Autodesk Inventor part; units mm, degrees
ref_plane "YZ Plane" through (0, 0, 0) normal (1, 0, 0) x (0, 1, 0)
ref_plane "XZ Plane" through (0, 0, 0) normal (0, 1, 0) x (-1, 0, 0)
ref_plane "XY Plane" through (0, 0, 0) normal (0, 0, 1) x (1, 0, 0)
sketch "스케치1" plane through (0, 0, 0) normal (0, 0, 1) x (1, 0, 0)
  line L0 (14.1048, -8.184) -> (-14.1048, -8.184)
  line L1 (-14.1048, -8.184) -> (-14.1048, 8.184)
  line L2 (-14.1048, 8.184) -> (14.1048, 8.184)
  line L3 (14.1048, 8.184) -> (14.1048, -8.184)
  line L4 (14.1048, -8.184) -> (-14.1048, 8.184) construction
  line L5 (-14.1048, -8.184) -> (14.1048, 8.184) construction
  point P0 (0, 0)
extrude "돌출1" add sketch "스케치1" along normal blind 20
sketch "스케치2" plane through (-14.1048, 8.184, 0) normal (0, 1, 0) x (1, 0, 0)
  line L0 (0, -20) -> (28.2096, -20)
  line L1 (28.2096, 0) -> (0, 0)
  line L2 (6.0629, -20) -> (28.2096, -20)
  line L3 (28.2096, -20) -> (28.2096, 0)
  line L4 (28.2096, 0) -> (6.0629, 0)
  line L5 (6.0629, 0) -> (6.0629, -20)
  point P0 (14.1048, 0)
extrude "돌출2" cut sketch "스케치2" against normal blind 8
sketch "스케치3" plane through (-14.1048, 0.184, 0) normal (0, 1, 0) x (1, 0, 0)
  line L0 (6.0629, -20) -> (6.0629, 0)
  line L1 (28.2096, 0) -> (28.2096, -20)
  line L2 (6.0629, -5.1676) -> (28.2096, -5.1676)
  line L3 (28.2096, -5.1676) -> (28.2096, -14.7078)
  line L4 (28.2096, -14.7078) -> (6.0629, -14.7078)
  line L5 (6.0629, -14.7078) -> (6.0629, -5.1676)
  point P0 (14.1048, 0)
extrude "돌출3" cut sketch "스케치3" against normal blind 4
sketch "스케치4" plane through (-8.0419, 8.184, 20) normal (1, 0, 0) x (0, 0, -1)
  point P0 (20, -8.184)
sketch "스케치5" plane through (-8.0419, 8.184, 20) normal (1, 0, 0) x (0, 0, -1)
  line L0 (5.2922, -8) -> (5.2922, -12)
  line L1 (5.2922, -12) -> (14.8018, -12)
  line L2 (14.8018, -12) -> (14.8018, -4.7287)
  line L3 (14.8018, -4.7287) -> (5.2922, -4.7287)
  line L4 (5.2922, -4.7287) -> (5.2922, -12)
  point P0 (20, -8.184)
extrude "돌출4" cut sketch "스케치5" against normal blind 10
chamfer "모따기1" distance 4 angle 45 1 edges at (-11.0733, 8.184, 20)
chamfer "모따기2" distance 4 angle 45 1 edges at (-11.0733, 8.184, 0)
chamfer "모따기3" distance 3 angle 45 1 edges at (14.1048, -4, 20)
chamfer "모따기4" distance 3 angle 45 1 edges at (14.1048, -4, 0)
chamfer "모따기5" distance 3 angle 45 1 edges at (-14.1048, -8.184, 10)
properties part number "240503_3Dsketch10"
Model file for the job. Use its own axes, mm. A direction names the side the tool comes from. Coordinates: 2 decimals unless noted, no trailing zeros. Write each loop counter-clockwise with the first axis right and the second up, starting at its lowest first coordinate (ties: lowest second). Pieces come first, ordered by that corner, then holes. Notation, with made-up numbers: (-19, 29) - (-13, 29) arc R13 cw to (-13, 39) - close; hole circle Ø6 at (-15.5, 65.25). An arc over 180 degrees is marked (long way). One line per question, with ' | ' between items. Start each with the question number.
Q1. Pin check, flat tips, straight feed: pin 1 (1 mm diameter, centred on x = 6, y = -1.5, fed in from -Z); pin 2 (3.5 mm diameter, centred on y = 4, z = 7.5, fed in from +X); pin 3 (6 mm diameter, centred on x = 2, z = 18, fed in from +Y); pin 4 (4 mm diameter, centred on x = -7.5, y = 6.5, fed in from -Z). Stop position of each tip, or through.
Q2. Cut at C-C, the plane z = 11.5. List the corners of the cut face in (x, y).
Q3. 3-axis set-ups, long thin cutter, end or side, ignore diameter. For faces 4 (the face through (12.584, -4.059, 1.479)), 5 (the face through (3, -2, 5.168)), 6 (the face through (0, -3.816, 10)), 7 (the face through (3, 0.184, 17)): which of +Z, -Z, +X, -X, +Y, -Y reach the whole face in a straight line?
Q4. Drill centre lines: line 1 (Z direction, x = 3.5, y = -2.75); line 2 (Y direction, x = 5.25, z = 19); line 3 (Y direction, x = -3.25, z = 6.25). Where is each one in solid material? Low to high. Write a range as [from, to].
Q5. Cut at B-B, the plane x = -8.5. List the corners of the cut face in (y, z), then the cut area to 3 significant figures.
Q6. Cut at D-D, the plane z = 4.5. List the corners of the cut face in (x, y), then the cut area to 3 significant figures.
Q7. Pull direction Y, two halves, no side cores. Call faces 1 (the face through (-11, 8.184, 10)), 2 (the face through (-2, -3, 0)), 3 (the face through (-3, -1, 14.708)): pulls with the +Y half, pulls with the -Y half, needs draft (parallel to the pull), parting line crosses it, or undercut.
Answer below:
1) pin 1: z = 0 | pin 2: x = -8.04 | pin 3: y = 0.18 | pin 4: z = 0.39
2) outline: (-14.1, -5.18) - (-11.1, -8.18) - (14.1, -8.18) - (14.1, -3.82) - (-14.1, -3.82) - close; (-14.1, 3.46) - (-8.04, 3.46) - (-8.04, 8.18) - (-14.1, 8.18) - close
3) face 4: -Z, +X, +Y, -Y | face 5: +X, +Y | face 6: +X, -X | face 7: +Z, -Z, +X, +Y
4) line 1: [0, 5.17], [14.71, 20] | line 2: [-8.18, 0.18] | line 3: [-8.18, -3.82]
5) outline: (-8.18, 0) - (4.18, 0) - (8.18, 4) - (8.18, 16) - (4.18, 20) - (-8.18, 20) - close; hole (-3.82, 5.2) - (3.46, 5.2) - (3.46, 14.71) - (-3.82, 14.71) - close | area: 242 mm^2
6) outline: (-14.1, -5.18) - (-11.1, -8.18) - (14.1, -8.18) - (14.1, 0.18) - (-8.04, 0.18) - (-8.04, 8.18) - (-14.1, 8.18) - close | area: 280 mm^2
7) face 1: pulls with the +Y half | face 2: needs draft | face 3: undercut
